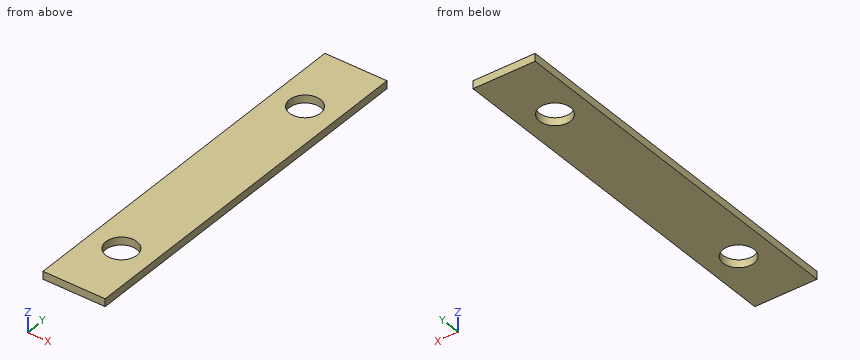
from build123d import *

# Parameters (mm, degrees)
F0_W     = 25.4
F0_H     = 152.4
F1_DEPTH = 3.175
F3_D     = 12.7
F3_DEPTH = 25.4
F3_TIP   = 3.8154649308
F4_D     = 12.7
F4_DEPTH = 25.4
F4_TIP   = 3.8154649308


with BuildPart() as f1:
    # F0 (on Top) → F1 (new body)
    with BuildSketch(Plane.XY):
        Rectangle(F0_W, F0_H)
    extrude(amount=F1_DEPTH)

    # F3
    with Locations(Plane(origin=(0, 0, 0), x_dir=(1, 0, 0), z_dir=(0, 0, -1))):
        with Locations((0, -48.6843948386)):
            Hole(F3_D / 2, depth=F3_DEPTH)
            with Locations((0, 0, -(F3_DEPTH + F3_TIP / 2))):  # 118° drill point
                Cone(0, F3_D / 2, F3_TIP, mode=Mode.SUBTRACT)

    # F4
    with Locations(Plane(origin=(0, 0, 0), x_dir=(1, 0, 0), z_dir=(0, 0, -1))):
        with Locations((0, 50.612956785)):
            Hole(F4_D / 2, depth=F4_DEPTH)
            with Locations((0, 0, -(F4_DEPTH + F4_TIP / 2))):  # 118° drill point
                Cone(0, F4_D / 2, F4_TIP, mode=Mode.SUBTRACT)


solid = f1.part
The listing builds one solid part. Answer for the finished solid, in the listing's coordinates (mm). Give positions to 0.01 mm unless a question says otherwise; leave off trailing zeros. Write each loop counter-clockwise with the first axis right and the second up, starting at its lowest first coordinate (ties: lowest second). Pieces come first, ordered by that corner, then holes.
1) Section B-B (y = 53) is taken. Write down the section's boundary in (x, z) (3 decimals).
2) Section A-A (x = 0) is taken. Write down the section's boundary in (y, z) (3 decimals), and give its area (3 significant figures).
3) Section C-C (z = 1.9) is taken. Write down the section's boundary in (x, y), and give its area (3 significant figures).
4) Find the intervals of material crossed by L1, parallel to Y at x = 0, z = 1.45; L2, parallel to Y at x = 0.75, z = 2.3; L3, parallel to X at y = -54, z = 2.9, in increasing order.
Response:
1. outline: (-12.7, 0) - (-4.658, 0) - (-4.658, 3.175) - (-12.7, 3.175) - close; (4.658, 0) - (12.7, 0) - (12.7, 3.175) - (4.658, 3.175) - close
2. outline: (-76.2, 0) - (-56.963, 0) - (-56.963, 3.175) - (-76.2, 3.175) - close; (-44.263, 0) - (42.334, 0) - (42.334, 3.175) - (-44.263, 3.175) - close; (55.034, 0) - (76.2, 0) - (76.2, 3.175) - (55.034, 3.175) - close
2. area: 403 mm2
3. outline: (-12.7, -76.2) - (12.7, -76.2) - (12.7, 76.2) - (-12.7, 76.2) - close; hole circle Ø12.7 at (0, -50.61); hole circle Ø12.7 at (0, 48.68)
3. area: 3,620 mm2
4. L1: y = -76.2 to -56.96, -44.26 to 42.33, 55.03 to 76.2
4. L2: y = -76.2 to -56.92, -44.31 to 42.38, 54.99 to 76.2
4. L3: x = -12.7 to -5.37, 5.37 to 12.7
